```python
from build123d import *

# Parameters (mm, degrees)
BOSS_EXTRUDE1_DEPTH = 5.334


with BuildPart() as part:
    # Sketch1 → Boss-Extrude1 (new body)
    with BuildSketch(Plane.XY):
        Polygon((0, 0), (0, 19.05), (5.334, 19.05), (5.334, 31.75), (0, 31.75), (0, 47.625), (5.334, 47.625), (5.334, 60.325), (0, 60.325), (0, 76.2), (-50.8, 0), (-41.275, 0), (-41.275, -5.08), (-28.575, -5.08), (-28.575, 0), align=None)
    extrude(amount=BOSS_EXTRUDE1_DEPTH)


solid = part.part
```
Could you check a few things on this model? Use its own coordinates, in mm. A direction names the side the tool comes from. Give positions to 0.01 mm unless a question says otherwise; leave off trailing zeros. Loops run counter-clockwise (first coordinate to the right, second up) from the corner with the lowest first, then second, coordinate; pieces in that order, holes last. Notation, with made-up numbers: (-4, -14.5) - (24, -14.5) arc R14 ccw to (24, 10.5) - close; hole circle Ø11 at (77.25, 10.25). An arc over 180 degrees is marked (long way). Answer in a Markdown table with one row per item. Add a question column.
Q1. If we section it at A-A (x = 1.5): List the corners of the cut face in (y, z) for me (3 decimals).
Q2. If we section it at D-D (x = -43): List the corners of the cut face in (y, z) for me.
Q3. Which directions (+Z, -Z, +X, -X, +Y, -Y) give clear straight access to the entire face, cutting with the end or side of a thin tool? Please do faces 5 (the face through (3, 19.05, 3)), 6 (the face through (3, 60.325, 3)), 7 (the face through (-41.275, -3, 3)).
Q4. We'd pull the mould along Y, two halves only. Please class faces 1 (the face through (-46, 0, 3)), 2 (the face through (3, 47.625, 3)), 3 (the face through (3, 31.75, 3)), 4 (the face through (-17, 18, 0)): +Y half, -Y half, draft (parallel to the pull), parting line (faces both ways), or undercut.
Q5. Please list where these lines run through material, in increasing order: L1, parallel to Y at x = 1, z = 4.35 (3 decimals); L2, parallel to Y at x = -14, z = 3.2; L3, parallel to Y at x = -18, z = 4.2. Write a range as from..to.
Q6. If we section it at C-C (y = 28.5): List the corners of the cut face in (x, z) for me.
Q7. For pin 1 (2.5 mm diameter, centred on x = -19.5, z = 2.5, fed in from -Y); pin 2 (2.5 mm diameter, centred on x = 3.5, z = 2, fed in from -Y); pin 3 (1.6 mm diameter, centred on x = 2.5, z = 4, fed in from +Y) (3 decimals), each with a flat end and sliding along its axis, tell me the tip position at first contact or that it passes through.
Q8. If we section it at B-B (z = 3.05): List the corners of the cut face in (x, y) for me (3 decimals).
The answers:
| question | item | result |
|---|---|---|
| 1 | outline | (19.05, 0) - (31.75, 0) - (31.75, 5.334) - (19.05, 5.334) - close; (47.625, 0) - (60.325, 0) - (60.325, 5.334) - (47.625, 5.334) - close |
| 2 | outline | (0, 0) - (11.7, 0) - (11.7, 5.33) - (0, 5.33) - close |
| 3 | face 5 | +Z, -Z, +X, -Y |
| 3 | face 6 | +Z, -Z, +X, +Y |
| 3 | face 7 | +Z, -Z, -X, -Y |
| 4 | face 1 | -Y half |
| 4 | face 2 | undercut |
| 4 | face 3 | undercut |
| 4 | face 4 | draft |
| 5 | L1 | y = 19.05..31.75, 47.625..60.325 |
| 5 | L2 | y = 0..55.2 |
| 5 | L3 | y = 0..49.2 |
| 6 | outline | (-31.8, 0) - (5.33, 0) - (5.33, 5.33) - (-31.8, 5.33) - close |
| 7 | pin 1 | stops at y = 0 |
| 7 | pin 2 | stops at y = 19.05 |
| 7 | pin 3 | stops at y = 60.325 |
| 8 | outline | (-50.8, 0) - (-41.275, 0) - (-41.275, -5.08) - (-28.575, -5.08) - (-28.575, 0) - (0, 0) - (0, 19.05) - (5.334, 19.05) - (5.334, 31.75) - (0, 31.75) - (0, 47.625) - (5.334, 47.625) - (5.334, 60.325) - (0, 60.325) - (0, 76.2) - close |
